Autodesk Inventor part; units mm, degrees
ref_plane "YZ Plane" through (0, 0, 0) normal (1, 0, 0) x (0, 1, 0)
ref_plane "XZ Plane" through (0, 0, 0) normal (0, 1, 0) x (-1, 0, 0)
ref_plane "XY Plane" through (0, 0, 0) normal (0, 0, 1) x (1, 0, 0)
sketch "Boceto1" plane through (0, 0, 0) normal (0, 0, 1) x (1, 0, 0)
  line L0 (-4.7609, 13.4664) -> (-4.7609, -16.5336)
  line L1 (-4.7609, -16.5336) -> (0.4391, -16.5336)
  line L2 (0.4391, -16.5336) -> (0.4391, -14.8936)
  line L3 (-0.9609, -15.1336) -> (-3.3609, -15.1336)
  line L4 (-3.3609, -15.1336) -> (-3.3609, -3.0336)
  line L5 (-2.8609, -2.5336) -> (17.5391, -2.5336)
  line L6 (18.0391, -3.0336) -> (18.0391, -7.2336)
  line L7 (18.0391, -7.2336) -> (14.2391, -7.2336)
  line L8 (14.2391, -7.2336) -> (14.2391, -8.8736)
  line L9 (14.9333, -9.8836) -> (15.6391, -9.8836)
  line L10 (15.6391, -9.8836) -> (15.6391, -8.6336)
  line L11 (15.6391, -8.6336) -> (18.0391, -8.6336)
  line L12 (18.0391, -8.6336) -> (18.0391, -15.1336)
  line L13 (18.0391, -15.1336) -> (15.6391, -15.1336)
  line L14 (15.6391, -15.1336) -> (15.6391, -13.8836)
  line L15 (15.6391, -13.8836) -> (14.9333, -13.8836)
  line L16 (14.2391, -14.8936) -> (14.2391, -16.5336)
  line L17 (14.2391, -16.5336) -> (19.4391, -16.5336)
  line L18 (19.4391, -16.5336) -> (19.4391, 13.4664)
  line L19 (-3.3609, 13.4664) -> (-3.3609, -0.6336)
  line L20 (18.0391, -0.6336) -> (18.0391, 13.4664)
  line L21 (7.3391, 11.7517) -> (7.3391, -2.5336) construction
  arc A0 (6.2391, 3.4216) -> (8.4391, 3.4216) centre (7.3391, 1.5164) ccw
  line L22 (-8.4881, 13.4664) -> (24.4446, 13.4664) construction
  line L23 (4.9522, 1.2664) -> (5.1534, 1.2664)
  line L24 (4.9522, 1.7664) -> (5.1534, 1.7664)
  line L25 (-2.8609, -1.1336) -> (3.8304, -1.1336)
  line L26 (10.8478, -1.1336) -> (17.5391, -1.1336)
  line L27 (4.0797, 1.5164) -> (9.7739, 1.5164) construction
  line L28 (9.726, 1.2664) -> (9.5249, 1.2664)
  line L29 (9.726, 1.7664) -> (9.5249, 1.7664)
  line L30 (7.5891, -0.8706) -> (7.5891, -0.6694)
  line L31 (7.0891, -0.8706) -> (7.0891, -0.6694)
  arc A1 (7.0891, -0.8706) -> (7.5891, -0.8706) centre (7.3391, 1.5164) ccw
  arc A2 (9.726, 1.2664) -> (9.726, 1.7664) centre (7.3391, 1.5164) ccw
  arc A3 (4.9522, 1.7664) -> (4.9522, 1.2664) centre (7.3391, 1.5164) ccw
  circle A4 centre (7.3391, 1.5164) radius 2.4 construction
  line L32 (6.2391, 4.9599) -> (6.2391, 3.4216)
  line L33 (8.4391, 4.9599) -> (8.4391, 3.4216)
  arc A5 (10.4214, -0.3724) -> (8.4391, 4.9599) centre (7.3391, 1.5164) ccw
  arc A6 (6.2391, 4.9599) -> (4.2568, -0.3724) centre (7.3391, 1.5164) ccw
  line L34 (-0.9609, -15.1336) -> (-0.9609, -13.8836)
  line L35 (-0.9609, -13.8836) -> (-0.2551, -13.8836)
  line L36 (-0.2551, -13.8836) -> (0.4391, -14.8936)
  line L37 (14.2391, -8.8736) -> (14.9333, -9.8836)
  line L38 (14.2391, -14.8936) -> (14.9333, -13.8836)
  arc A7 (-2.8609, -2.5336) -> (-3.3609, -3.0336) centre (-2.8609, -3.0336) ccw
  arc A8 (-3.3609, -0.6336) -> (-2.8609, -1.1336) centre (-2.8609, -0.6336) ccw
  arc A9 (17.5391, -1.1336) -> (18.0391, -0.6336) centre (17.5391, -0.6336) ccw
  arc A10 (18.0391, -3.0336) -> (17.5391, -2.5336) centre (17.5391, -3.0336) ccw
  arc A11 (3.8304, -1.1336) -> (4.2568, -0.3724) centre (3.8304, -0.6336) ccw
  arc A12 (10.4214, -0.3724) -> (10.8478, -1.1336) centre (10.8478, -0.6336) ccw
  line L39 (-4.7609, 13.4664) -> (-4.7609, 43.4664)
  line L40 (-4.7609, 43.4664) -> (0.4391, 43.4664)
  line L41 (0.4391, 43.4664) -> (0.4391, 41.8264)
  line L42 (-0.9609, 42.0664) -> (-3.3609, 42.0664)
  line L43 (-3.3609, 42.0664) -> (-3.3609, 29.9664)
  line L44 (-2.8609, 29.4664) -> (17.5391, 29.4664)
  line L45 (18.0391, 29.9664) -> (18.0391, 34.1664)
  line L46 (18.0391, 34.1664) -> (14.2391, 34.1664)
  line L47 (14.2391, 34.1664) -> (14.2391, 35.8064)
  line L48 (14.9333, 36.8164) -> (15.6391, 36.8164)
  line L49 (15.6391, 36.8164) -> (15.6391, 35.5664)
  line L50 (15.6391, 35.5664) -> (18.0391, 35.5664)
  line L51 (18.0391, 35.5664) -> (18.0391, 42.0664)
  line L52 (18.0391, 42.0664) -> (15.6391, 42.0664)
  line L53 (15.6391, 42.0664) -> (15.6391, 40.8164)
  line L54 (15.6391, 40.8164) -> (14.9333, 40.8164)
  line L55 (14.2391, 41.8264) -> (14.2391, 43.4664)
  line L56 (14.2391, 43.4664) -> (19.4391, 43.4664)
  line L57 (19.4391, 43.4664) -> (19.4391, 13.4664)
  line L58 (-3.3609, 13.4664) -> (-3.3609, 27.5664)
  line L59 (18.0391, 27.5664) -> (18.0391, 13.4664)
  line L60 (7.3391, 15.181) -> (7.3391, 29.4664) construction
  arc A13 (8.4391, 23.5111) -> (6.2391, 23.5111) centre (7.3391, 25.4164) ccw
  line L61 (4.9522, 25.6664) -> (5.1534, 25.6664)
  line L62 (4.9522, 25.1664) -> (5.1534, 25.1664)
  line L63 (-2.8609, 28.0664) -> (3.8304, 28.0664)
  line L64 (10.8478, 28.0664) -> (17.5391, 28.0664)
  line L65 (4.0797, 25.4164) -> (9.7739, 25.4164) construction
  line L66 (9.726, 25.6664) -> (9.5249, 25.6664)
  line L67 (9.726, 25.1664) -> (9.5249, 25.1664)
  line L68 (7.5891, 27.8033) -> (7.5891, 27.6021)
  line L69 (7.0891, 27.8033) -> (7.0891, 27.6021)
  arc A14 (7.5891, 27.8033) -> (7.0891, 27.8033) centre (7.3391, 25.4164) ccw
  arc A15 (9.726, 25.1664) -> (9.726, 25.6664) centre (7.3391, 25.4164) ccw
  arc A16 (4.9522, 25.6664) -> (4.9522, 25.1664) centre (7.3391, 25.4164) ccw
  circle A17 centre (7.3391, 25.4164) radius 2.4 construction
  line L70 (6.2391, 21.9728) -> (6.2391, 23.5111)
  line L71 (8.4391, 21.9728) -> (8.4391, 23.5111)
  arc A18 (8.4391, 21.9728) -> (10.4214, 27.3051) centre (7.3391, 25.4164) ccw
  arc A19 (4.2568, 27.3051) -> (6.2391, 21.9728) centre (7.3391, 25.4164) ccw
  line L72 (-0.9609, 42.0664) -> (-0.9609, 40.8164)
  line L73 (-0.9609, 40.8164) -> (-0.2551, 40.8164)
  line L74 (-0.2551, 40.8164) -> (0.4391, 41.8264)
  line L75 (14.2391, 35.8064) -> (14.9333, 36.8164)
  line L76 (14.2391, 41.8264) -> (14.9333, 40.8164)
  arc A20 (-3.3609, 29.9664) -> (-2.8609, 29.4664) centre (-2.8609, 29.9664) ccw
  arc A21 (-2.8609, 28.0664) -> (-3.3609, 27.5664) centre (-2.8609, 27.5664) ccw
  arc A22 (18.0391, 27.5664) -> (17.5391, 28.0664) centre (17.5391, 27.5664) ccw
  arc A23 (17.5391, 29.4664) -> (18.0391, 29.9664) centre (17.5391, 29.9664) ccw
  arc A24 (4.2568, 27.3051) -> (3.8304, 28.0664) centre (3.8304, 27.5664) ccw
  arc A25 (10.8478, 28.0664) -> (10.4214, 27.3051) centre (10.8478, 27.5664) ccw
  point P0 (4.8803, -1.1336)
  point P1 (9.7979, -1.1336)
  point P2 (7.3391, -2.5336)
  point P3 (18.0391, -11.8836)
  point P4 (4.8803, 28.0664)
  point P5 (9.7979, 28.0664)
  point P6 (7.3391, 29.4664)
  point P7 (18.0391, 38.8164)
  dimension "d0" = 1.4
  dimension "d1" = 1.4
  dimension "d2" = 1.4
  dimension "d3" = 1.4
  dimension "d4" = 1.4
  dimension "d5" = 1.4
  dimension "d6" = 1.4
  dimension "d7" = 1.4
  dimension "d8" = 1.4
  dimension "d9" = 1.4
  dimension "d12" = 4.4
  dimension "d19" = 0.5
  dimension "d22" = 4.05
  dimension "d24" = 0.25
  dimension "d25" = 0.25
  dimension "d26" = 0.5
  dimension "d30" = 0.5
  dimension "d32" = 4.8
  dimension "d35" = 1.1
  dimension "d36" = 2.2
  dimension "d37" = 1.415
  dimension "d38" = 1.415
  dimension "d39" = 0.2
  dimension "d40" = 0.2
  dimension "d42" = 30
  dimension "d43" = 14
  dimension "d44" = 4
  dimension "d45" = 9.3
  dimension "d46" = 6.5
  dimension "d47" = 24.2
  dimension "d48" = 5.2
  dimension "d49" = 1.4
  dimension "d50" = 5.2
  dimension "d51" = 13.8
  dimension "d52" = 21.4
  dimension "d53" = 0.2
  dimension "d55" = 0.2
  dimension "d56" = 0.25
  dimension "d57" = 0.2
  dimension "d58" = 1.4
  dimension "d62" = 1.4
  dimension "d63" = 2.65
  dimension "d64" = 1.64
  dimension "d65" = 34.5
  dimension "d66" = 2
  dimension "d67" = 2
  dimension "d68" = 2.4
  dimension "d69" = 3.01
  dimension "d70" = 6.02
  dimension "d71" = 34.5
  dimension "d72" = 111
  dimension "d74" = 0.7058
  dimension "d75" = 0.7058
  dimension "d82" = 9.6652
  dimension "d83" = 25.6354
  dimension "d84" = 15.3594
  dimension "d86" = 0.5
  dimension "d87" = 0.5
  dimension "d88" = 60
  dimension "d89" = 30.6
extrude "Extrusión1" add sketch "Boceto1" against normal blind 602
properties part number "SP40-04A TRAVESAÑO CENTRAL" material "Aluminio"
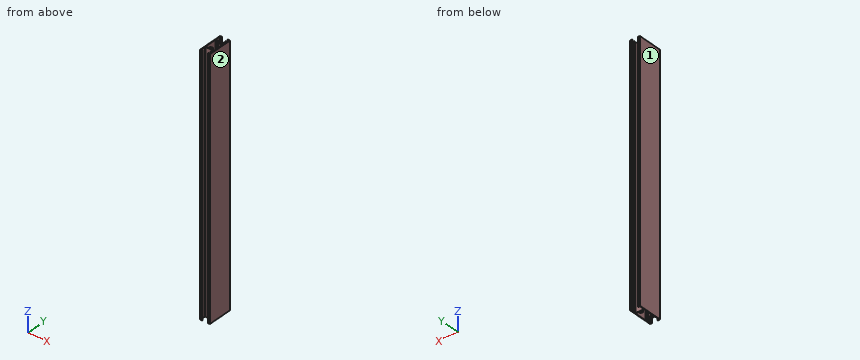
Geometry check sheet. Reference: the model listing, model coordinates, mm. Face numbers are marked on the shaded views. Give positions to 0.01 mm unless a question says otherwise; leave off trailing zeros. Loops run counter-clockwise (first coordinate to the right, second up) from the corner with the lowest first, then second, coordinate; pieces in that order, holes last. Notation, with made-up numbers: (-22, 85) -> (-8, 85) arc R17 ccw to (-8, 100) -> close; hole circle Ø4 at (10, 57.5). An arc over 180 degrees is marked (long way). Answer in a Markdown table with one row per item. Add a question column.
1) Gauge pin test, flat ends, axial feed: P1, Ø3, axis at x = -2, y = 20.5, coming from the +Z side; P2, Ø2, axis at x = 11, z = -253.5, coming from the -Y side; P3, Ø1.5, axis at x = 4.5, z = -495.5, coming from the +Y side. Record the tip position at first contact, or that the pin passes through.
2) Draft check along X on the marked faces 1 and 2. Enter one of: pulls with the +X half, pulls with the -X half, needs draft (parallel to the pull), parting line crosses it, or undercut.
3) Material ranges on probe 1 along Y at (x, z) = (17, -80); probe 2 along Y at (x, z) = (-2, -310.5); probe 3 along X at (y, z) = (40.5, -547.5), recorded low to high. Write a range as from..to.
4) Cross-section at A-A on y = 11. Record the boundary of the cut face in (x, z).
Outcome:
| question | item | result |
|---|---|---|
| 1 | P1 | stops at z = 0 |
| 1 | P2 | stops at y = -2.53 |
| 1 | P3 | stops at y = 29.47 |
| 2 | face 1 | pulls with the -X half |
| 2 | face 2 | pulls with the +X half |
| 3 | probe 1 | y = -16.53..-15.13, -8.63..-7.23, -2.53..-1.13, 28.07..29.47, 34.17..35.57, 42.07..43.47 |
| 3 | probe 2 | y = -16.53..-15.13, -2.53..-1.13, 28.07..29.47, 42.07..43.47 |
| 3 | probe 3 | x = -4.76..-3.36, 18.04..19.44 |
| 4 | outline | (-4.76, -602) -> (-3.36, -602) -> (-3.36, 0) -> (-4.76, 0) -> close; (18.04, -602) -> (19.44, -602) -> (19.44, 0) -> (18.04, 0) -> close |
